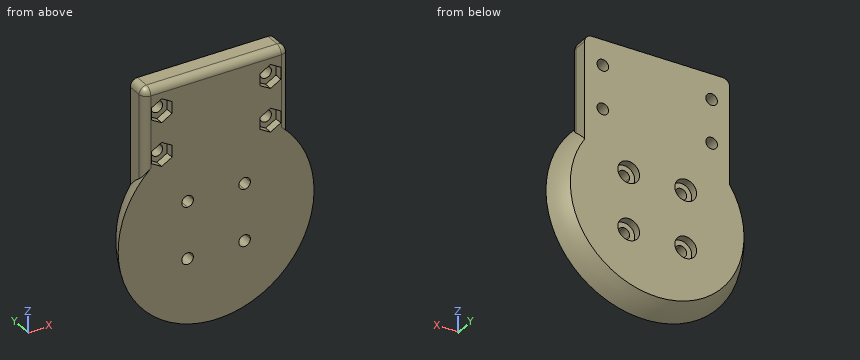
from build123d import *

# Parameters (mm, degrees)
SKETCH_15_W          = 40
SKETCH_15_H          = 18.792360098
EXTRUDE_5_DEPTH      = 42
CUT_EXTRUDE_9_DEPTH  = 77.440518039
CUT_EXTRUDE_10_DEPTH = 51.289163843
SKETCH_18_R          = 3
CUT_EXTRUDE_11_DEPTH = 2.2
SKETCH_19_R          = 1.6
CUT_EXTRUDE_12_DEPTH = 51.289163843
CUT_EXTRUDE_13_DEPTH = 2.2
FILLET_2_R           = 2


with BuildPart() as part:
    # 草图14 → 旋转4 (revolve)
    with BuildSketch(Plane.XY):
        with BuildLine():
            Line((0, 18.792360098), (0, 0))
            Line((0, 0), (27, 0))
            ThreePointArc((27, 0), (16.448045462, 13.631796387), (0, 18.792360098))
        make_face()
    revolve(axis=Axis((0, 18.792360098, 0), (0, -1, 0)))

    # 草图15 → 凸台-拉伸5 (add)
    with BuildSketch(Plane.XY):
        with Locations((0, 9.396180049)):
            Rectangle(SKETCH_15_W, SKETCH_15_H)
    extrude(amount=EXTRUDE_5_DEPTH)

    # 草图16 → 切除-拉伸9 (cut, through all)
    with BuildSketch(Plane.XY.offset(42)):
        Polygon((-20, 6), (0, 6), (20, 6), (20, 18.792360098), (-20, 18.792360098), align=None)
        Polygon((20, 18.792360098), (20, 6), (23.937418407, 6), (23.937418407, 21.459034266), (-28.897937851, 21.459034266), (-28.897937851, 6), (-20, 6), (-20, 18.792360098), align=None)
    extrude(amount=-CUT_EXTRUDE_9_DEPTH, mode=Mode.SUBTRACT)

    # 草图17 → 切除-拉伸10 (cut, through all)
    with BuildSketch(Plane(origin=(0, 6, 0), x_dir=(1, 0, 0), z_dir=(0, 1, 0))):
        with BuildLine():
            Line((-7.86, 6.26), (-7.86, 7.86))
            Line((-7.86, 7.86), (-6.26, 7.86))
            ThreePointArc((-6.26, 7.86), (-8.99137085, 8.99137085), (-7.86, 6.26))
        make_face()
        with BuildLine():
            Line((-6.26, 7.86), (-7.86, 7.86))
            Line((-7.86, 7.86), (-7.86, 6.26))
            ThreePointArc((-7.86, 6.26), (-6.72862915, 6.72862915), (-6.26, 7.86))
        make_face()
        with BuildLine():
            ThreePointArc((9.46, 7.86), (7.86, 9.46), (6.26, 7.86))
            Line((6.26, 7.86), (7.86, 7.86))
            Line((7.86, 7.86), (7.86, 6.26))
            ThreePointArc((7.86, 6.26), (8.99137085, 6.72862915), (9.46, 7.86))
        make_face()
        with BuildLine():
            Line((7.86, 7.86), (6.26, 7.86))
            ThreePointArc((6.26, 7.86), (6.72862915, 6.72862915), (7.86, 6.26))
            Line((7.86, 6.26), (7.86, 7.86))
        make_face()
        with BuildLine():
            ThreePointArc((9.46, -7.86), (8.99137085, -6.72862915), (7.86, -6.26))
            Line((7.86, -6.26), (7.86, -7.86))
            Line((7.86, -7.86), (6.26, -7.86))
            ThreePointArc((6.26, -7.86), (7.86, -9.46), (9.46, -7.86))
        make_face()
        with BuildLine():
            Line((7.86, -7.86), (7.86, -6.26))
            ThreePointArc((7.86, -6.26), (6.72862915, -6.72862915), (6.26, -7.86))
            Line((6.26, -7.86), (7.86, -7.86))
        make_face()
        with BuildLine():
            ThreePointArc((-6.26, -7.86), (-6.72862915, -6.72862915), (-7.86, -6.26))
            Line((-7.86, -6.26), (-7.86, -7.86))
            Line((-7.86, -7.86), (-6.26, -7.86))
        make_face()
        with BuildLine():
            Line((-7.86, -7.86), (-7.86, -6.26))
            ThreePointArc((-7.86, -6.26), (-8.99137085, -8.99137085), (-6.26, -7.86))
            Line((-6.26, -7.86), (-7.86, -7.86))
        make_face()
    extrude(amount=-CUT_EXTRUDE_10_DEPTH, mode=Mode.SUBTRACT)

    # 草图18 → 切除-拉伸11 (cut)
    with BuildSketch(Plane(origin=(0, 6, 0), x_dir=(1, 0, 0), z_dir=(0, 1, 0))):
        with Locations(Location((7.86, 7.86, 0), (0, 0, 180))):
            Circle(SKETCH_18_R)
        with Locations(Location((7.86, -7.86, 0), (0, 0, 180))):
            Circle(SKETCH_18_R)
        with Locations(Location((-7.86, -7.86, 0), (0, 0, 180))):
            Circle(SKETCH_18_R)
        with Locations(Location((-7.86, 7.86, 0), (0, 0, 180))):
            Circle(SKETCH_18_R)
    extrude(amount=-CUT_EXTRUDE_11_DEPTH, mode=Mode.SUBTRACT)

    # 草图19 → 切除-拉伸12 (cut, through all)
    with BuildSketch(Plane(origin=(0, 6, 0), x_dir=(1, 0, 0), z_dir=(0, 1, 0))):
        with Locations(Location((15, -23.002515628, 0), (0, 0, 180))):
            Circle(SKETCH_19_R)
        with Locations(Location((-15, -23.002515628, 0), (0, 0, 180))):
            Circle(SKETCH_19_R)
        with Locations(Location((-15, -35.002515628, 0), (0, 0, 180))):
            Circle(SKETCH_19_R)
        with Locations(Location((15, -35.002515628, 0), (0, 0, 180))):
            Circle(SKETCH_19_R)
    extrude(amount=-CUT_EXTRUDE_12_DEPTH, mode=Mode.SUBTRACT)

    # 草图20 → 切除-拉伸13 (cut)
    with BuildSketch(Plane.XZ):
        Polygon((-15, 31.711619093), (-12.15, 33.35706736), (-12.15, 36.647963895), (-15, 38.293412162), (-17.85, 36.647963895), (-17.85, 33.35706736), align=None)
        Polygon((15, 31.711619093), (17.85, 33.35706736), (17.85, 36.647963895), (15, 38.293412162), (12.15, 36.647963895), (12.15, 33.35706736), align=None)
        Polygon((-15, 19.711619093), (-12.15, 21.35706736), (-12.15, 24.647963895), (-15, 26.293412162), (-17.85, 24.647963895), (-17.85, 21.35706736), align=None)
        Polygon((15, 19.711619093), (17.85, 21.35706736), (17.85, 24.647963895), (15, 26.293412162), (12.15, 24.647963895), (12.15, 21.35706736), align=None)
    extrude(amount=-CUT_EXTRUDE_13_DEPTH, mode=Mode.SUBTRACT)

    # 圆角2
    fillet_2_edges = [part.edges().sort_by_distance(p)[0] for p in [
        (20, 0, 30.069178574),
        (-20, 0, 30.069178574),
        (0, 0, 42),
        (-20, 3, 42),
        (20, 3, 42),
    ]]
    fillet(fillet_2_edges, radius=FILLET_2_R)


solid = part.part
Verification items for the finished model (mm, model axes). Give positions to 0.01 mm unless a question says otherwise; leave off trailing zeros. Write each loop counter-clockwise with the first axis right and the second up, starting at its lowest first coordinate (ties: lowest second). Pieces come first, ordered by that corner, then holes. Notation, with made-up numbers: (61, 34.25) -> (86, 34.25) arc R27 cw to (86, 73.25) -> close; hole circle Ø11 at (44, -10.5). An arc over 180 degrees is marked (long way). Use CSV: the item, a comma, the result in double quotes.
(1) Sectioned sample at C-C (x = 21). Record the cut outline in (y, z).
Derived:
outline,"(0, -16.97) arc R19.7 ccw to (6, -11.49) -> (6, 11.49) arc R19.7 ccw to (0, 16.97) -> close"
(2) Sectioned sample at A-A (y = 5). Give the number of separate pieces and of enclosed holes in the cut face, plus the area to 3 significant figures.
Derived:
separate pieces,"1"
enclosed holes,"8"
area,"2,570 mm^2"
(3) Material ranges on L1, parallel to Z at x = 14, y = 2.5; L2, parallel to Z at x = 15.5, y = 2; L3, parallel to X at y = 0.5, z = 23.5, recorded low to high.
Derived:
L1,"z = -21.83 to 21.75, 24.25 to 33.75, 36.25 to 42"
L2,"z = -21.09 to 20, 26 to 32, 38 to 42"
L3,"x = -19.32 to -17.85, -12.15 to 12.15, 17.85 to 19.32"
(4) Go/stop test with flat-tipped pins: pin 1 (3 mm diameter, centred on y = 0.5, z = 26, fed in from -X); pin 2 (2.5 mm diameter, centred on y = 1.5, z = 34.5, fed in from +X); pin 3 (3 mm diameter, centred on y = 3.5, z = 11.5, fed in from +X). Record where each tip stops, or that it passes through.
Derived:
pin 1,"stops at x = -20"
pin 2,"stops at x = 20"
pin 3,"stops at x = 23.78"
(5) Sectioned sample at B-B (z = 30). Record the cut outline in (x, y).
Derived:
outline,"(-20, 2) arc R2 ccw to (-18, 0) -> (18, 0) arc R2 ccw to (20, 2) -> (20, 6) -> (-20, 6) -> close"
